Geometry: final body of the model. Coordinates: model frame, mm. Coordinates: 2 decimals unless noted, no trailing zeros. Order: outer loops, then holes, each group sorted by start corner. A loop starts at its lowest first (then second) coordinate and runs counter-clockwise, first axis right, second up. Notation, with made-up numbers: (58.5, -13) -> (85.5, -13) arc R16 cw to (85.5, -8) -> close; hole circle Ø7 at (77.25, 13.5). An arc over 180 degrees is marked (long way). Use one line per item in the form item = value.
```python
from build123d import *

# Parameters (mm, degrees)
ESBO_O1_R                = 2
RESSALTO_EXTRUS_O1_DEPTH = 2.5


with BuildPart() as part:
    # Esboço1 → Ressalto-extrusão1 (new body)
    with BuildSketch(Plane(origin=(0, 0, 0), x_dir=(1, 0, 0), z_dir=(0, 1, 0))):
        with BuildLine():
            Line((11.040621421, -63.022227155), (11.975083319, -63.022227155))
            ThreePointArc((11.975083319, -63.022227155), (13.927517872, -62.083636556), (14.413923052, -59.972626609))
            add(Edge.make_bspline(
                [(14.628150734, 61.977772845), (9.961904295, 43.145041124), (5.80089976, 0.158887719), (10.360032358, -41.983580286), (14.413923052, -59.972626609)],
                knots=[0, 0, 0, 0, 0.486126784, 0.972253568, 0.972253568, 0.972253568, 0.972253568], degree=3))
            Line((14.628150734, 61.977772845), (11.221984798, 61.977772845))
            ThreePointArc((11.221984798, 61.977772845), (-1.551940129, 57.366952224), (-8.43603741, 45.660457041))
            add(Edge.make_bspline(
                [(-8.43603741, 45.660457041), (-10.928367674, 32.356496924), (-14.334494692, 2.382887461), (-11.960473063, -29.417729259), (-8.595648838, -46.819185188)],
                knots=[0.126810365, 0.126810365, 0.126810365, 0.126810365, 0.438278248, 0.866480416, 0.866480416, 0.866480416, 0.866480416], degree=3))
            ThreePointArc((-8.595648838, -46.819185188), (-1.688495582, -58.448489837), (11.040621421, -63.022227155))
        make_face()
        with Locations(Location((5.00152215, 16.977772845, 0), (0, 0, 270))):
            Circle(ESBO_O1_R, mode=Mode.SUBTRACT)
        with Locations(Location((5.125334517, -5.021878755, 0), (0, 0, 270))):
            Circle(ESBO_O1_R, mode=Mode.SUBTRACT)
    extrude(amount=RESSALTO_EXTRUS_O1_DEPTH)


solid = part.part
```
1) Contact query for flat-ended pins moving along their axis: P1, Ø1.5, axis at y = 0.5, z = 16.5, coming from the -X side; P2, Ø1.5, axis at x = -1.5, y = 2, coming from the +Z side. Output: stop coordinate, or through.
Results found:
P1 = -12.46
P2 = 59.18
2) Section B-B, the plane y = 2. Give the number of separate pieces and of enclosed holes in the cut face, and give its area (3 significant figures).
Results found:
separate_pieces = 1
enclosed_holes = 2
area = 2,420 mm2
3) Section A-A, the plane x = -5.75. Output: boundary loops of the cut face in (y, z).
Results found:
outline = (0, -52.56) -> (2.5, -52.56) -> (2.5, 53.89) -> (0, 53.89) -> close
4) Material intervals for probe 1 along Z at (x, y) = (5.75, 1.45); probe 2 along Z at (x, y) = (6.5, 1.1); probe 3 along X at (y, z) = (1.15, 6), sorted ascending. Write a range as from..to.
Results found:
probe_1 = -61.21..-18.83, -15.12..3.12, 6.92..62.31
probe_2 = -61.41..-18.3, -15.65..3.57, 6.47..62.5
probe_3 = -12.84..3.38, 6.87..8.08
5) Pull-direction query (Z, two-part tool) for faces 1 (the cylindrical face through (-1.4, 1.23, -57.49)), 2 (the cylindrical face through (5.73, 1.23, 6.93)), 3 (the flat face through (0, 2.5, 0)), 4 (the cylindrical face through (5.6, 1.23, -15.07)); classes: released by +Z, released by -Z, zero draft, split by the parting line, or undercut.
Results found:
face_1 = released by -Z
face_2 = undercut
face_3 = zero draft
face_4 = undercut
